from build123d import *

# Parameters (mm, degrees)
F0_R     = 10
F0_R_2   = 6.15
F1_DEPTH = 25
F2_R     = 10
F3_DEPTH = 38
F5_DEPTH = 5
F6_R     = 3.05
F7_DEPTH = 50
F8_SIZE  = 0.8
F9_SIZE  = 0.4
F10_SIZE = 0.4


with BuildPart() as f1:
    # F0 (on Top) → F1 (new body)
    with BuildSketch(Plane.XY):
        Circle(F0_R)
        Circle(F0_R_2, mode=Mode.SUBTRACT)
    extrude(amount=F1_DEPTH)

    # F2 (on face) → F3 (join)
    with BuildSketch(Plane.XY.offset(25)):
        Circle(F2_R)
    extrude(amount=F3_DEPTH)

    # F4 (on face) → F5 (cut)
    with BuildSketch(Plane(origin=(0, 0, 25), x_dir=(1, 0, 0), z_dir=(0, 0, -1))):
        Polygon((-2.915619, -5.05), (2.915619, -5.05), (5.831238, 0), (2.915619, 5.05), (-2.915619, 5.05), (-5.831238, 0), align=None)
    extrude(amount=-F5_DEPTH, mode=Mode.SUBTRACT)

    # F6 (on face) → F7 (cut)
    with BuildSketch(Plane(origin=(0, 0, 30), x_dir=(1, 0, 0), z_dir=(0, 0, -1))):
        Circle(F6_R)
    extrude(amount=-F7_DEPTH, mode=Mode.SUBTRACT)

    # F8
    f8_edges = [f1.edges().sort_by_distance(p)[0] for p in [
        (-10, 0, 0),
        (-10, 0, 63),
    ]]
    chamfer(f8_edges, length=F8_SIZE)

    # F9
    f9_edges = [f1.edges().sort_by_distance(p)[0] for p in [
        (-3.05, 0, 63),
    ]]
    chamfer(f9_edges, length=F9_SIZE)

    # F10
    f10_edges = [f1.edges().sort_by_distance(p)[0] for p in [
        (-6.15, 0, 0),
    ]]
    chamfer(f10_edges, length=F10_SIZE)


solid = f1.part
Design review of the part built by this model. Coordinates are the model's own, in mm. A direction names the side the tool comes from. Coordinates: 2 decimals unless noted, no trailing zeros. Loops run counter-clockwise (first coordinate to the right, second up) from the corner with the lowest first, then second, coordinate; pieces in that order, holes last. Notation, with made-up numbers: M -38.75,0.25 L -2.75,0.25 A22 cw -2.75,37.25 Z; hole C 1,39 d3. An arc over 180 degrees is marked long. Answer as CSV lines item,"result".
Item 1: For probe 1 along Y at (x, z) = (0, 6); probe 2 along Y at (x, z) = (0, 43); probe 3 along Z at (x, y) = (-4.75, -0.25), list the stretches that pass through material, from the lowest coordinate up.
Answer list:
probe 1,"-10 to -6.15, 6.15 to 10"
probe 2,"-10 to -3.05, 3.05 to 10"
probe 3,"30 to 63"
Item 2: The part is to be moulded in two halves that separate along Y. For faces 1 (the face through (-2.17, -9.76, 31.07)), 2 (the face through (0, -4, 63)), 3 (the face through (-5, 2, 25)), say which applies: pulls with the +Y half, pulls with the -Y half, needs draft (parallel to the pull), parting line crosses it, or undercut.
Answer list:
face 1,"parting line crosses it"
face 2,"needs draft"
face 3,"undercut"
Item 3: Add section A-A on x = 0. State the section outline as (y, z) points, plus the area to 3 significant figures.
Answer list:
outline,"M -10,0.8 L -9.2,0 L -6.55,0 L -6.15,0.4 L -6.15,25 L -5.05,25 L -5.05,30 L -3.05,30 L -3.05,62.6 L -3.45,63 L -9.2,63 L -10,62.2 Z; M 3.05,30 L 5.05,30 L 5.05,25 L 6.15,25 L 6.15,0.4 L 6.55,0 L 9.2,0 L 10,0.8 L 10,62.2 L 9.2,63 L 3.45,63 L 3.05,62.6 Z"
area,"699 mm²"
Item 4: Add section C-C on z = 17. State the section outline as (x, y) points.
Answer list:
outline,"C 0,0 d20; hole C 0,0 d12.3"
Item 5: Machinability: for faces 4 (the face through (4.353, 2.56, 27.465)), 5 (the face through (-3.047, -0.134, 46.072)), which of the approach directions +Z, -Z, +X, -X, +Y, -Y give a long, thin tool a straight path to every point of the face, cutting with its end or side? Answer none if there is none.
Answer list:
face 4,"-Z"
face 5,"+Z, -Z"
Item 6: For P1, Ø11, axis at x = 0, y = 0, coming from the -Z side; P2, Ø3, axis at y = -6, z = 11.5, coming from the +X side; P3, Ø2, axis at y = -6.5, z = 21, coming from the -X side; P4, Ø5, axis at x = 0, y = 0, coming from the +Z side, all flat-tipped, find the tip position at first contact; note any pin that passes through.
Answer list:
P1,"z = 25"
P2,"x = 8.93"
P3,"x = -8.35"
P4,"through"
Item 7: Add section B-B on z = 59. State the section outline as (x, y) points, plus the area to 3 significant figures.
Answer list:
outline,"C 0,0 d20; hole C 0,0 d6.1"
area,"285 mm²"
